Answer from the drawing. Dimensions are ordinates in mm from the lowest x, y and z of the part. Round coordinates to 2 decimals unless told otherwise and drop trailing zeros. Write each loop counter-clockwise with the first axis right and the second up, starting at its lowest first coordinate (ties: lowest second). Pieces come first, ordered by that corner, then holes. Notation, with made-up numbers: M -26.5,59.25 L 0.5,59.25 A15 cw 0.5,68.25 Z; hole C 5,-34.5 d4. An arc over 180 degrees is marked long. Answer as CSV lines item,"result". Start each with the question number.
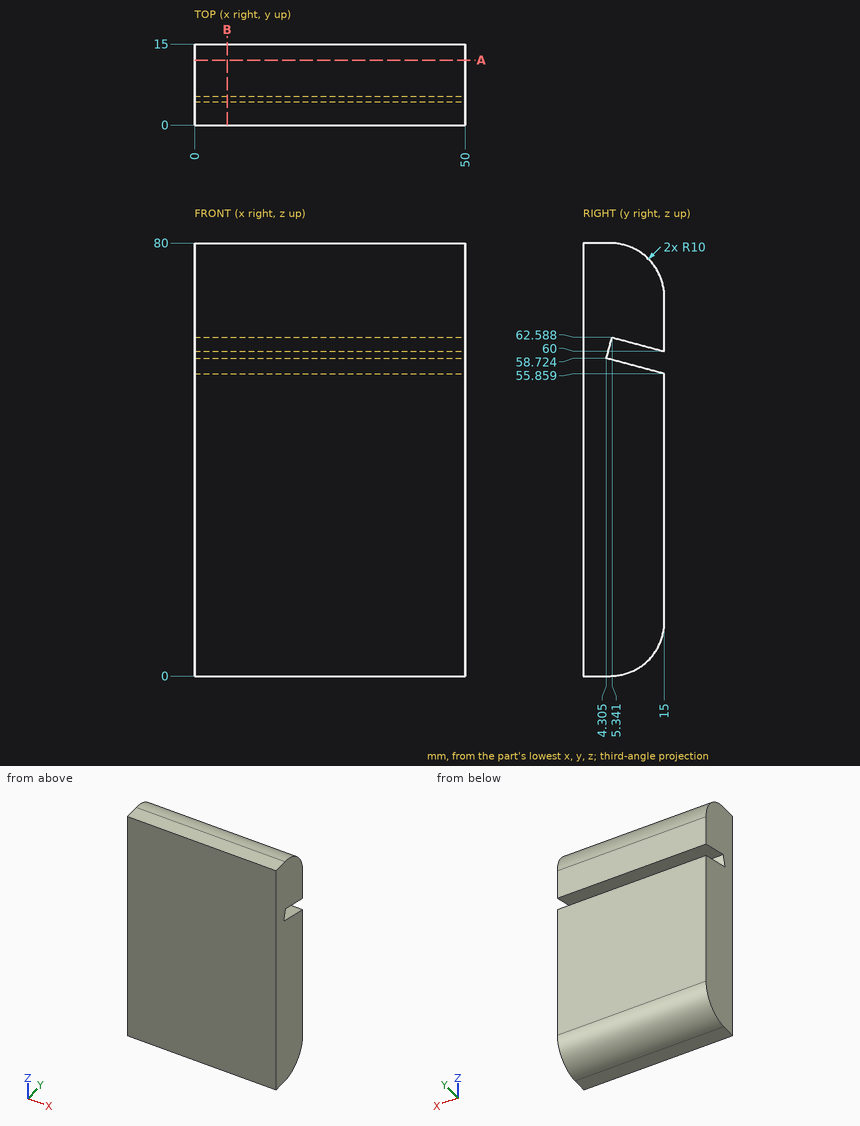
Q1. Find section A-A (y = 12). Determine the outline of the cut face in (x, z).
Q2. Find section B-B (x = 6). Determine the outline of the cut face in (y, z) (1 decimal).
Q3. Straight lines are drawn through the part: L1, parallel to Z at x = 4.5, y = 12.75 (1 decimal); L2, parallel to Z at x = 11, y = 7.25 (1 decimal); L3, parallel to Y at x = 24, z = 4.5. For each, find the intervals that lie inside material, in ascending order.
Reported:
1,outline,"M 0,2.86 L 50,2.86 L 50,56.66 L 0,56.66 Z; M 0,60.8 L 50,60.8 L 50,77.14 L 0,77.14 Z"
2,outline,"M 0,0 L 5,0 A10 ccw 15,10 L 15,55.9 L 4.3,58.7 L 5.3,62.6 L 15,60 L 15,70 A10 ccw 5,80 L 0,80 Z"
3,L1,"z = 3.7 to 56.5, 60.6 to 76.3"
3,L2,"z = 0.3 to 57.9, 62.1 to 79.7"
3,L3,"y = 0 to 13.35"
